Here's how the part is built. I have some questions about the finished solid (model axes, mm). A direction names the side the tool comes from. Give positions to 0.01 mm unless a question says otherwise; leave off trailing zeros. Write each loop counter-clockwise with the first axis right and the second up, starting at its lowest first coordinate (ties: lowest second). Pieces come first, ordered by that corner, then holes. Notation, with made-up numbers: (45.25, 79.25) -> (90.25, 79.25) arc R21 cw to (90.25, 98.25) -> close; hole circle Ø7 at (5, 76.5). An arc over 180 degrees is marked (long way). Put each result on its own line as item: value. Start each with the question number.
Autodesk Fusion 360 part; units mm, degrees
sketch "Sketch1" plane through (0, 0, 0) normal (0, 0, 1) x (1, 0, 0)
  line L0 (2.55, 1.55) -> (-2.55, -1.55) construction
  line L1 (2.55, 1.55) -> (-2.55, -1.55) construction
  line L2 (-2.55, 1.55) -> (-2.55, -1.55)
  circle A0 centre (0, 0) radius 4
  line L3 (-2.55, 1.55) -> (2.55, -1.55) construction
  line L4 (-2.55, -1.55) -> (2.55, -1.55)
  line L5 (2.55, 1.55) -> (-2.55, 1.55)
  line L6 (2.55, 1.55) -> (-2.55, -1.55) construction
  line L7 (-2.55, 1.55) -> (2.55, -1.55) construction
  line L8 (-2.55, 1.55) -> (2.55, -1.55) construction
  circle A1 centre (0, 0) radius 2.55
  line L9 (2.55, -1.55) -> (2.55, 1.55)
  line L10 (-10, 10) -> (10, 10)
  line L11 (10, 10) -> (10, -10)
  line L12 (10, -10) -> (-10, -10)
  line L13 (-10, -10) -> (-10, 10)
  circle A2 centre (-7, 7) radius 1.5
  line L14 (0, 10) -> (0, 7.5)
  circle A3 centre (7, 7) radius 1.5
  line L15 (-10, 0) -> (-8.5, 0)
  circle A4 centre (-7, -7) radius 1.5
  circle A5 centre (7, -7) radius 1.5
  dimension "d1" = 5.1
  dimension "d2" = 5.1
  dimension "d3" = 3.1
  dimension "d4" = 8
  dimension "d5" = 5.1
  dimension "d6" = 5.1
  dimension "d7" = 20
  dimension "d8" = 20
  dimension "d9" = 3
extrude "Extrude1" add sketch "Sketch1" along normal blind 10 contours L2 L5 A1 | L2 L4 A1 | L5 A1 | L4 A1 | L5 A1 L9 | L4 A1 L9 | A0 makes body 1
extrude "Extrude2" add sketch "Sketch1" against normal blind 3 separate body contours L10 L11 L12 L13 makes body 2
extrude "Extrude3" add sketch "Sketch1" against normal blind 3 contours L2 L5 A1 | L2 L4 A1 | L4 L5 A1 | L5 A1 | L4 A1 | L5 A1 L9 | L4 A1 L9 | A0 bodies 1 2
1) I want a section at C-C, the plane z = -2. Write out the boundary of the cut face in (x, y), and give its area (3 significant figures).
2) I want a section at A-A, the plane x = 7. Write out the boundary of the cut face in (y, z), and give its area (3 significant figures).
3) Thinking about a two-plate mould opening in X: for faces 1 (the cylindrical face through (5.8, -7.9, -1.5)), 2 (the flat face through (10, 0, -1)), 3 (the flat face through (-10, 0, -1)), 4 (the flat face through (0, -2, 10)), which applies, released by +X, released by -X, zero draft, split by the parting line, or undercut?
4) I'm going to push flat-ended pins straight in: pin 1 Ø4 at (x, y) = (7, -7) entering from -Z; pin 2 Ø3 at (y, z) = (-3, 4) entering from -X; pin 3 Ø1.6 at (x, y) = (-1, -0.5) entering from +Z; pin 4 Ø1.2 at (x, z) = (0.5, 4) entering from +Y. Where does each tip first touch, or does it pass through?
5) Which directions (+Z, -Z, +X, -X, +Y, -Y) give clear straight access to the entire face, cutting with the end or side of a thin tool? Please do faces 5 (the flat face through (0, 0, 0)), 6 (the cylindrical face through (5.8, 6.1, -1.5)).
6) I need wall thicknesses on probe 1 along Y at (x, z) = (7, -1.2); probe 2 along Z at (x, y) = (-2.5, -4.5); probe 3 along X at (y, z) = (-1, 1.25). Which ranges of each line are inside material? Lowest first, please.
7) I want a section at D-D, the plane y = 0. Write out the boundary of the cut face in (x, z).
Established:
1. outline: (-10, -10) -> (10, -10) -> (10, 10) -> (-10, 10) -> close; hole circle Ø3 at (-7, -7); hole circle Ø3 at (-7, 7); hole circle Ø3 at (7, -7); hole circle Ø3 at (7, 7)
1. area: 372 mm2
2. outline: (-10, -3) -> (-8.5, -3) -> (-8.5, 0) -> (-10, 0) -> close; (-5.5, -3) -> (5.5, -3) -> (5.5, 0) -> (-5.5, 0) -> close; (8.5, -3) -> (10, -3) -> (10, 0) -> (8.5, 0) -> close
2. area: 42.0 mm2
3. face 1: undercut
3. face 2: released by +X
3. face 3: released by -X
3. face 4: zero draft
4. pin 1: stops at z = -3
4. pin 2: stops at x = -3.71
4. pin 3: stops at z = 0
4. pin 4: stops at y = 4
5. face 5: +Z
5. face 6: +Z, -Z
6. probe 1: y = -10 to -8.5, -5.5 to 5.5, 8.5 to 10
6. probe 2: z = -3 to 0
6. probe 3: x = -3.87 to -2.35, 2.35 to 3.87
7. outline: (-10, -3) -> (10, -3) -> (10, 0) -> (4, 0) -> (4, 10) -> (2.55, 10) -> (2.55, 0) -> (-2.55, 0) -> (-2.55, 10) -> (-4, 10) -> (-4, 0) -> (-10, 0) -> close
